Verification items for this drawing (mm, ordinates from the low corner). Round coordinates to 2 decimals unless told otherwise and drop trailing zeros. Order: outer loops, then holes, each group sorted by start corner. A loop starts at its lowest first (then second) coordinate and runs counter-clockwise, first axis right, second up. Notation, with made-up numbers: (-36, 23) -> (-17, 23) arc R15 ccw to (-17, 42) -> close; hole circle Ø11 at (-37, 12.25). An arc over 180 degrees is marked (long way). Put each result on its own line as item: value.
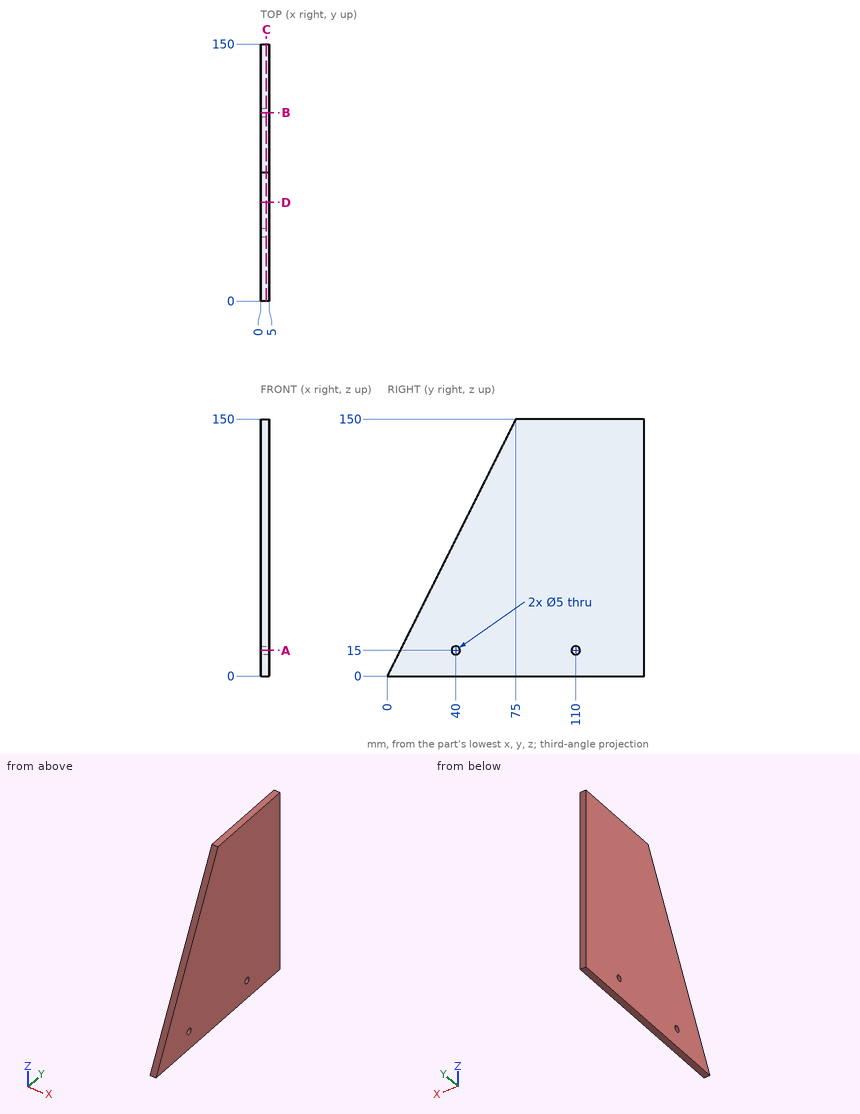
Item 1: Material ranges on L1, parallel to Y at x = 3.7, z = 15; L2, parallel to Y at x = 3, z = 75; L3, parallel to Y at x = 1.3, z = 73, recorded low to high. Write a range as [from, to].
Check sheet entries:
L1: y = [7.5, 37.5], [42.5, 107.5], [112.5, 150]
L2: y = [37.5, 150]
L3: y = [36.5, 150]
Item 2: Gauge pin test, flat end, axial feed: pin 1 Ø3 at (x, z) = (3.5, 126) entering from -Y. Record the tip position at first contact, or that the pin passes through.
Check sheet entries:
pin 1: stops at y = 62.25
Item 3: Section check B-B on y = 110. Record the boundary of the cut face in (x, z), then the cut area to 3 significant figures.
Check sheet entries:
outline: (0, 0) -> (5, 0) -> (5, 12.5) -> (0, 12.5) -> close; (0, 17.5) -> (5, 17.5) -> (5, 150) -> (0, 150) -> close
area: 725 mm^2
Item 4: Section check C-C on x = 3.3. Record the boundary of the cut face in (y, z).
Check sheet entries:
outline: (0, 0) -> (150, 0) -> (150, 150) -> (75, 150) -> close; hole circle Ø5 at (40, 15); hole circle Ø5 at (110, 15)
Item 5: Section check A-A on z = 15. Record the boundary of the cut face in (x, y), then the cut area to 4 significant figures.
Check sheet entries:
outline: (0, 7.5) -> (5, 7.5) -> (5, 37.5) -> (0, 37.5) -> close; (0, 42.5) -> (5, 42.5) -> (5, 107.5) -> (0, 107.5) -> close; (0, 112.5) -> (5, 112.5) -> (5, 150) -> (0, 150) -> close
area: 662.5 mm^2
Item 6: Section check D-D on y = 57.5. Record the boundary of the cut face in (x, z), then the cut area to 3 significant figures.
Check sheet entries:
outline: (0, 0) -> (5, 0) -> (5, 115) -> (0, 115) -> close
area: 575 mm^2
